Source: CAD feature listing. Evaluate the final solid. Frame: model axes, mm. A direction names the side the tool comes from. Round coordinates to 2 decimals unless told otherwise and drop trailing zeros. Order: outer loops, then holes, each group sorted by start corner. A loop starts at its lowest first (then second) coordinate and runs counter-clockwise, first axis right, second up.
```python
from build123d import *

# Parameters (mm, degrees)
SKETCH1_W              = 15
SKETCH1_H              = 6
MAIN_BODY_DEPTH        = 5
SKETCH3_R              = 1.25
GRIN_HOLE_DEPTH        = 4
SKETCH2_R              = 0.795
MAGNET_HOLES_DEPTH     = 1
SET_SCREW_INDENT_DEPTH = 6
SKETCH5_R              = 0.5
CUT_EXTRUDE1_DEPTH     = 2


with BuildPart() as part:
    # Sketch1 → Main Body (new body)
    with BuildSketch(Plane(origin=(0, 0, 0), x_dir=(1, 0, 0), z_dir=(0, 1, 0))):
        Rectangle(SKETCH1_W, SKETCH1_H)
    extrude(amount=MAIN_BODY_DEPTH)

    # Sketch3 → GRIN Hole (cut)
    with BuildSketch(Plane.XZ):
        with Locations((-4.5, 0)):
            Circle(SKETCH3_R)
    extrude(amount=-GRIN_HOLE_DEPTH, mode=Mode.SUBTRACT)

    # Sketch2 → Magnet Holes (cut)
    with BuildSketch(Plane.XZ):
        with Locations((-6.25, -1.875)):
            Circle(SKETCH2_R)
        with Locations((-6.25, 1.875)):
            Circle(SKETCH2_R)
        with Locations((-1.5, 0)):
            Circle(SKETCH2_R)
    extrude(amount=-MAGNET_HOLES_DEPTH, mode=Mode.SUBTRACT)

    # Sketch4 → Set Screw Indent (cut, through all)
    with BuildSketch(Plane.XZ):
        Polygon((7.058045095, -3), (7.5, -1.895112738), (7.5, -3), align=None)
    extrude(amount=-SET_SCREW_INDENT_DEPTH, mode=Mode.SUBTRACT)

    # Sketch5 → Cut-Extrude1 (cut)
    with BuildSketch(Plane.XZ):
        with Locations((-2, -2)):
            Circle(SKETCH5_R)
    extrude(amount=-CUT_EXTRUDE1_DEPTH, mode=Mode.SUBTRACT)


solid = part.part
```
1. Pull-direction query (Z, two-part tool) for faces 3 (the face through (-2.5, 1, -2)), 4 (the face through (-6.88, 0.49, -2.36)), 5 (the face through (0, 0, 0)), 6 (the face through (7.276, 2.465, -2.455)); classes: released by +Z, released by -Z, zero draft, split by the parting line, or undercut.
2. Section D-D on z = 0. Return loops of the section in (x, y) (3 decimals).
3. First-contact query: pin 1 (2 mm diameter, centred on x = -4.5, z = 0, fed in from -Y); pin 2 (1 mm diameter, centred on x = -1.5, z = 0, fed in from -Y). Flat tips, straight axial feed; report the tip coordinate or a pass-through.
4. Section B-B on x = -3.5. Return loops of the section in (y, z), plus the area to 3 significant figures.
5. Section A-A on y = 1.2. Return loops of the section in (x, z), plus the area to 3 significant figures.
6. Line query: line 1 along Z through (x, y) = (-6.25, 0.55); line 2 along X through (y, z) = (3, -0.1); line 3 along Z through (x, y) = (-2, 1.05). Output: solid intervals per line, ascending.
7. Access query for faces 1 (the face through (-1.133, 0.493, -0.705)), 2 (the face through (-7.5, 2, 0)). Directions: +Z, -Z, +X, -X, +Y, -Y. A direction counts if a zero-diameter tool reaches every point of the face in a straight line with its end or side. Return the directions, or none.
8. Section C-C on y = 3.05. Return loops of the section in (x, z).
Result:
1. face 3: undercut
1. face 4: undercut
1. face 5: zero draft
1. face 6: released by -Z
2. outline: (-7.5, 0) - (-5.75, 0) - (-5.75, 4) - (-3.25, 4) - (-3.25, 0) - (-2.295, 0) - (-2.295, 1) - (-0.705, 1) - (-0.705, 0) - (7.5, 0) - (7.5, 5) - (-7.5, 5) - close
3. pin 1: stops at y = 4
3. pin 2: stops at y = 1
4. outline: (0, -3) - (5, -3) - (5, 3) - (0, 3) - (0, 0.75) - (4, 0.75) - (4, -0.75) - (0, -0.75) - close
4. area: 24.0 mm2
5. outline: (-7.5, -3) - (7.06, -3) - (7.5, -1.9) - (7.5, 3) - (-7.5, 3) - close; hole circle Ø2.5 at (-4.5, 0); hole circle Ø1 at (-2, -2)
5. area: 84.1 mm2
6. line 1: z = -3 to -2.67, -1.08 to 1.08, 2.67 to 3
6. line 2: x = -7.5 to -5.75, -3.25 to 7.5
6. line 3: z = -3 to -2.5, -1.5 to 3
7. face 1: -Y
7. face 2: +Z, -Z, -X, +Y, -Y
8. outline: (-7.5, -3) - (7.06, -3) - (7.5, -1.9) - (7.5, 3) - (-7.5, 3) - close; hole circle Ø2.5 at (-4.5, 0)
